Source: CAD feature listing. Evaluate the final solid. Frame: model axes, mm. Face numbers are marked on the shaded views. A direction names the side the tool comes from. Give positions to 0.01 mm unless a question says otherwise; leave off trailing zeros. Order: outer loops, then holes, each group sorted by start corner. A loop starts at its lowest first (then second) coordinate and runs counter-clockwise, first axis right, second up.
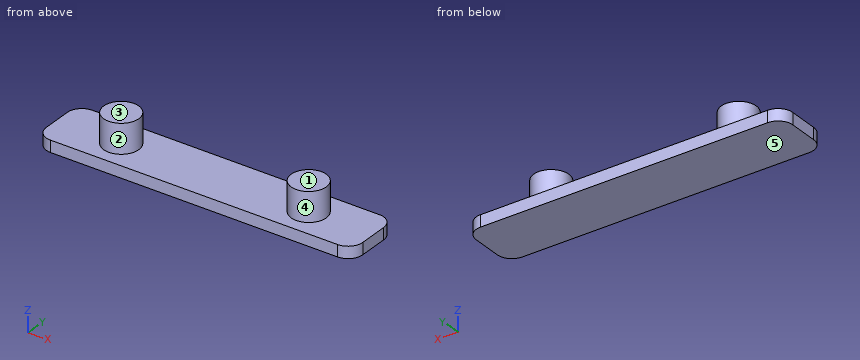
```python
from build123d import *

# Parameters (mm, degrees)
BOSS_EXTRUDE1_DEPTH = 2
SKETCH2_R           = 3
BOSS_EXTRUDE2_DEPTH = 5


with BuildPart() as part:
    # Sketch1 → Boss-Extrude1 (new body)
    with BuildSketch(Plane.XY):
        with BuildLine():
            Line((-5.313337951, 3.839414132), (43.686662049, 3.839414132))
            ThreePointArc((43.686662049, 3.839414132), (45.454429002, 3.107181085), (46.186662049, 1.339414132))
            Line((46.186662049, 1.339414132), (46.186662049, -3.660585868))
            ThreePointArc((46.186662049, -3.660585868), (45.454429002, -5.428352821), (43.686662049, -6.160585868))
            Line((43.686662049, -6.160585868), (-5.313337951, -6.160585868))
            ThreePointArc((-5.313337951, -6.160585868), (-7.081104904, -5.428352821), (-7.813337951, -3.660585868))
            Line((-7.813337951, -3.660585868), (-7.813337951, 1.339414132))
            ThreePointArc((-7.813337951, 1.339414132), (-7.081104904, 3.107181085), (-5.313337951, 3.839414132))
        make_face()
    extrude(amount=BOSS_EXTRUDE1_DEPTH)

    # Sketch2 → Boss-Extrude2 (add)
    with BuildSketch(Plane.XY.offset(2)):
        with Locations(Location((3.186662049, -1.160585868, 0), (0, 0, 180))):
            Circle(SKETCH2_R)
        with Locations(Location((35.186662049, -1.160585868, 0), (0, 0, 180))):
            Circle(SKETCH2_R)
    extrude(amount=BOSS_EXTRUDE2_DEPTH)


solid = part.part
```
1) Section query D-D, the plane y = -3. Return the cut outline in (x, z), and give its area (3 significant figures).
Report:
outline: (-7.81, 0) - (46.19, 0) - (46.19, 2) - (37.56, 2) - (37.56, 7) - (32.82, 7) - (32.82, 2) - (5.56, 2) - (5.56, 7) - (0.82, 7) - (0.82, 2) - (-7.81, 2) - close
area: 155 mm2
2) Material intervals for L1, parallel to Z at x = -4, y = 2; L2, parallel to X at y = 1, z = 5.75; L3, parallel to X at y = -3, z = 4.5, sorted ascending.
Report:
L1: z = 0 to 2
L2: x = 1.11 to 5.27, 33.11 to 37.27
L3: x = 0.82 to 5.56, 32.82 to 37.56
3) Draft query along Z for the marked faces 3, 4 and 5. Return one class per face: +Z half, -Z half, draft (parallel to the pull), parting line (faces both ways), or undercut.
Report:
face 3: +Z half
face 4: draft
face 5: -Z half
4) Reachability of the marked faces 1 and 2 from +Z, -Z, +X, -X, +Y, -Y: full face, straight path, thin tool, end or side. Return the list, or none.
Report:
face 1: +Z, +X, -X, +Y, -Y
face 2: +Z
5) Section query B-B, the plane y = 0. Return the cut outline in (x, z).
Report:
outline: (-7.81, 0) - (46.19, 0) - (46.19, 2) - (37.95, 2) - (37.95, 7) - (32.42, 7) - (32.42, 2) - (5.95, 2) - (5.95, 7) - (0.42, 7) - (0.42, 2) - (-7.81, 2) - close
6) Section query A-A, the plane z = 5.25. Return the cut outline in (x, y).
Report:
outline: circle Ø6 at (3.19, -1.16); circle Ø6 at (35.19, -1.16)
7) Section query C-C, the plane x = 31.5. Return the cut outline in (y, z), and give its area (3 significant figures).
Report:
outline: (-6.16, 0) - (3.84, 0) - (3.84, 2) - (-6.16, 2) - close
area: 20.0 mm2
8) Pin query (flat end, axial travel): pin 1 (1.5 mm diameter, centred on x = 22.5, y = 2, fed in from +Z); pin 2 (4 mm diameter, centred on x = 28, z = 4.5, fed in from -Y); pin 3 (2 mm diameter, centred on x = 32.5, z = 4.5, fed in from +Y). Return the tip coordinate at first contact, or that it passes through.
Report:
pin 1: stops at z = 2
pin 2: passes through
pin 3: stops at y = 1.32
